from build123d import *

# Parameters (mm, degrees)
RESSALTO_EXTRUS_O2_DEPTH = 9.2
ESBO_O5_R                = 2.15
CORTE_EXTRUS_O2_DEPTH    = 9.2
CHANFRO2_SIZE            = 0.3
SKETCH1_W                = 40
SKETCH1_H                = 3.972261678
BOSS_EXTRUDE1_DEPTH      = 88.9


with BuildPart() as part:
    # Esboço4 → Ressalto-extrusão2 (new body)
    with BuildSketch(Plane(origin=(0, 0, 0), x_dir=(1, 0, 0), z_dir=(0, 1, 0))):
        with BuildLine():
            Line((-19.2, 2.35), (-19.2, 1.65))
            ThreePointArc((-19.2, 1.65), (-19.170710678, 1.579289322), (-19.1, 1.55))
            Line((-19.1, 1.55), (-18.1, 1.55))
            ThreePointArc((-18.1, 1.55), (-18.029289322, 1.579289322), (-18, 1.65))
            Line((-18, 1.65), (-18, 2.35))
            ThreePointArc((-18, 2.35), (-17.970710678, 2.420710678), (-17.9, 2.45))
            Line((-17.9, 2.45), (-17.3, 2.45))
            ThreePointArc((-17.3, 2.45), (-17.229289322, 2.420710678), (-17.2, 2.35))
            Line((-17.2, 2.35), (-17.2, 1.65))
            ThreePointArc((-17.2, 1.65), (-17.170710678, 1.579289322), (-17.1, 1.55))
            Line((-17.1, 1.55), (-16.1, 1.55))
            ThreePointArc((-16.1, 1.55), (-16.029289322, 1.579289322), (-16, 1.65))
            Line((-16, 1.65), (-16, 2.35))
            ThreePointArc((-16, 2.35), (-15.970710678, 2.420710678), (-15.9, 2.45))
            Line((-15.9, 2.45), (-15.3, 2.45))
            ThreePointArc((-15.3, 2.45), (-15.229289322, 2.420710678), (-15.2, 2.35))
            Line((-15.2, 2.35), (-15.2, 1.65))
            ThreePointArc((-15.2, 1.65), (-15.170710678, 1.579289322), (-15.1, 1.55))
            Line((-15.1, 1.55), (-14.1, 1.55))
            ThreePointArc((-14.1, 1.55), (-14.029289322, 1.579289322), (-14, 1.65))
            Line((-14, 1.65), (-14, 2.35))
            ThreePointArc((-14, 2.35), (-13.970710678, 2.420710678), (-13.9, 2.45))
            Line((-13.9, 2.45), (-13.3, 2.45))
            ThreePointArc((-13.3, 2.45), (-13.229289322, 2.420710678), (-13.2, 2.35))
            Line((-13.2, 2.35), (-13.2, 1.65))
            ThreePointArc((-13.2, 1.65), (-13.170710678, 1.579289322), (-13.1, 1.55))
            Line((-13.1, 1.55), (-12.1, 1.55))
            ThreePointArc((-12.1, 1.55), (-12.029289322, 1.579289322), (-12, 1.65))
            Line((-12, 1.65), (-12, 2.35))
            ThreePointArc((-12, 2.35), (-11.970710678, 2.420710678), (-11.9, 2.45))
            Line((-11.9, 2.45), (-11.3, 2.45))
            ThreePointArc((-11.3, 2.45), (-11.229289322, 2.420710678), (-11.2, 2.35))
            Line((-11.2, 2.35), (-11.2, 1.65))
            ThreePointArc((-11.2, 1.65), (-11.170710678, 1.579289322), (-11.1, 1.55))
            Line((-11.1, 1.55), (-10.1, 1.55))
            ThreePointArc((-10.1, 1.55), (-10.029289322, 1.579289322), (-10, 1.65))
            Line((-10, 1.65), (-10, 2.35))
            ThreePointArc((-10, 2.35), (-9.970710678, 2.420710678), (-9.9, 2.45))
            Line((-9.9, 2.45), (-9.3, 2.45))
            ThreePointArc((-9.3, 2.45), (-9.229289322, 2.420710678), (-9.2, 2.35))
            Line((-9.2, 2.35), (-9.2, 1.65))
            ThreePointArc((-9.2, 1.65), (-9.170710678, 1.579289322), (-9.1, 1.55))
            Line((-9.1, 1.55), (-8.1, 1.55))
            ThreePointArc((-8.1, 1.55), (-8.029289322, 1.579289322), (-8, 1.65))
            Line((-8, 1.65), (-8, 2.35))
            ThreePointArc((-8, 2.35), (-7.970710678, 2.420710678), (-7.9, 2.45))
            Line((-7.9, 2.45), (-7.3, 2.45))
            ThreePointArc((-7.3, 2.45), (-7.229289322, 2.420710678), (-7.2, 2.35))
            Line((-7.2, 2.35), (-7.2, 1.65))
            ThreePointArc((-7.2, 1.65), (-7.170710678, 1.579289322), (-7.1, 1.55))
            Line((-7.1, 1.55), (7.1, 1.55))
            ThreePointArc((7.1, 1.55), (7.170710678, 1.579289322), (7.2, 1.65))
            Line((7.2, 1.65), (7.2, 2.35))
            ThreePointArc((7.2, 2.35), (7.229289322, 2.420710678), (7.3, 2.45))
            Line((7.3, 2.45), (7.9, 2.45))
            ThreePointArc((7.9, 2.45), (7.970710678, 2.420710678), (8, 2.35))
            Line((8, 2.35), (8, 1.65))
            ThreePointArc((8, 1.65), (8.029289322, 1.579289322), (8.1, 1.55))
            Line((8.1, 1.55), (9.1, 1.55))
            ThreePointArc((9.1, 1.55), (9.170710678, 1.579289322), (9.2, 1.65))
            Line((9.2, 1.65), (9.2, 2.35))
            ThreePointArc((9.2, 2.35), (9.229289322, 2.420710678), (9.3, 2.45))
            Line((9.3, 2.45), (9.9, 2.45))
            ThreePointArc((9.9, 2.45), (9.970710678, 2.420710678), (10, 2.35))
            Line((10, 2.35), (10, 1.65))
            ThreePointArc((10, 1.65), (10.029289322, 1.579289322), (10.1, 1.55))
            Line((10.1, 1.55), (11.1, 1.55))
            ThreePointArc((11.1, 1.55), (11.170710678, 1.579289322), (11.2, 1.65))
            Line((11.2, 1.65), (11.2, 2.35))
            ThreePointArc((11.2, 2.35), (11.229289322, 2.420710678), (11.3, 2.45))
            Line((11.3, 2.45), (11.9, 2.45))
            ThreePointArc((11.9, 2.45), (11.970710678, 2.420710678), (12, 2.35))
            Line((12, 2.35), (12, 1.65))
            ThreePointArc((12, 1.65), (12.029289322, 1.579289322), (12.1, 1.55))
            Line((12.1, 1.55), (13.1, 1.55))
            ThreePointArc((13.1, 1.55), (13.170710678, 1.579289322), (13.2, 1.65))
            Line((13.2, 1.65), (13.2, 2.35))
            ThreePointArc((13.2, 2.35), (13.229289322, 2.420710678), (13.3, 2.45))
            Line((13.3, 2.45), (13.9, 2.45))
            ThreePointArc((13.9, 2.45), (13.970710678, 2.420710678), (14, 2.35))
            Line((14, 2.35), (14, 1.65))
            ThreePointArc((14, 1.65), (14.029289322, 1.579289322), (14.1, 1.55))
            Line((14.1, 1.55), (15.1, 1.55))
            ThreePointArc((15.1, 1.55), (15.170710678, 1.579289322), (15.2, 1.65))
            Line((15.2, 1.65), (15.2, 2.35))
            ThreePointArc((15.2, 2.35), (15.229289322, 2.420710678), (15.3, 2.45))
            Line((15.3, 2.45), (15.9, 2.45))
            ThreePointArc((15.9, 2.45), (15.970710678, 2.420710678), (16, 2.35))
            Line((16, 2.35), (16, 1.65))
            ThreePointArc((16, 1.65), (16.029289322, 1.579289322), (16.1, 1.55))
            Line((16.1, 1.55), (17.1, 1.55))
            ThreePointArc((17.1, 1.55), (17.170710678, 1.579289322), (17.2, 1.65))
            Line((17.2, 1.65), (17.2, 2.35))
            ThreePointArc((17.2, 2.35), (17.229289322, 2.420710678), (17.3, 2.45))
            Line((17.3, 2.45), (17.9, 2.45))
            ThreePointArc((17.9, 2.45), (17.970710678, 2.420710678), (18, 2.35))
            Line((18, 2.35), (18, 1.65))
            ThreePointArc((18, 1.65), (18.029289322, 1.579289322), (18.1, 1.55))
            Line((18.1, 1.55), (19.1, 1.55))
            ThreePointArc((19.1, 1.55), (19.170710678, 1.579289322), (19.2, 1.65))
            Line((19.2, 1.65), (19.2, 2.35))
            ThreePointArc((19.2, 2.35), (19.229289322, 2.420710678), (19.3, 2.45))
            Line((19.3, 2.45), (19.9, 2.45))
            ThreePointArc((19.9, 2.45), (19.970710678, 2.420710678), (20, 2.35))
            Line((20, 2.35), (20, -2.45))
            Line((20, -2.45), (-20, -2.45))
            Line((-20, -2.45), (-20, 2.35))
            ThreePointArc((-20, 2.35), (-19.970710678, 2.420710678), (-19.9, 2.45))
            Line((-19.9, 2.45), (-19.3, 2.45))
            ThreePointArc((-19.3, 2.45), (-19.229289322, 2.420710678), (-19.2, 2.35))
        make_face()
    extrude(amount=RESSALTO_EXTRUS_O2_DEPTH)

    # Esboço5 → Corte-extrusão2 (cut)
    with BuildSketch(Plane(origin=(0, 0, -1.55), x_dir=(-1, 0, 0), z_dir=(0, 0, -1))):
        with Locations((0, 4.6)):
            Circle(ESBO_O5_R)
    extrude(amount=-CORTE_EXTRUS_O2_DEPTH, mode=Mode.SUBTRACT)

    # Chanfro2
    chanfro2_edges = [part.edges().sort_by_distance(p)[0] for p in [
        (2.15, 4.6, -1.55),
    ]]
    chamfer(chanfro2_edges, length=CHANFRO2_SIZE)

    # Sketch1 → Boss-Extrude1 (add)
    with BuildSketch(Plane.XZ):
        with Locations((0, 0.463869161)):
            Rectangle(SKETCH1_W, SKETCH1_H)
    extrude(amount=BOSS_EXTRUDE1_DEPTH)


solid = part.part
CAD build for the part. Positions are in the model's coordinates, mm. A direction names the side the tool comes from. Give positions to 0.01 mm unless a question says otherwise; leave off trailing zeros. Write each loop counter-clockwise with the first axis right and the second up, starting at its lowest first coordinate (ties: lowest second). Pieces come first, ordered by that corner, then holes. Notation, with made-up numbers: M 71,83 L 84,83 A20 ccw 84,106 Z; hole C 14,47.5 d8. An arc over 180 degrees is marked long. Put each result on its own line as item: value. Start each with the question number.
(1) Mould opens along X. For faces 1 (the face through (0.47, 2.5, 0.57)), 2 (the face through (-20, -39, 1)), 3 (the face through (0, -39, 2.45)) say: +X half, -X half, draft (parallel to the pull), parting line (faces both ways), or undercut.
(2) Band-saw the part on B-B, the plane y = -56.5. Write the cut outline in (x, z), and give its area (3 significant figures).
(3) Which spindle directions (+Z, -Z, +X, -X, +Y, -Y) get a long thin tool onto all of the face, cutting with end or side? Do faces 4 (the face through (0, -44, -1.522)), 5 (the face through (0, 9.2, 1)), 6 (the face through (-2, 7, -1.55)). Say none if no direction does.
(4) Flat gauge pins, fed straight in: pin 1 Ø8 at (x, y) = (-9, -40.5) entering from -Z; pin 2 Ø0.8 at (x, y) = (18.5, 4) entering from -Z; pin 3 Ø0.7 at (x, z) = (-7.5, -2) entering from -Y; pin 4 Ø2.5 at (x, y) = (0, 4.6) entering from -Z. Where does each tip first touch, or does it go through?
(5) Probe L1, parallel to Y at x = 0, z = 1.1; L2, parallel to Z at x = 16, y = -66.5; L3, parallel to X at y = 5, z = 1.9. List the from-to ranges inside material, lowest first.
Response values:
1. face 1: undercut
1. face 2: -X half
1. face 3: draft
2. outline: M -20,-1.52 L 20,-1.52 L 20,2.45 L -20,2.45 Z
2. area: 159 mm2
3. face 4: -Z, +X, -X, -Y
3. face 5: +Z, -Z, +X, -X, +Y
3. face 6: -Z, +Y, -Y
4. pin 1: stops at z = -1.52
4. pin 2: stops at z = -1.55
4. pin 3: stops at y = 0
4. pin 4: passes through
5. L1: y = -88.9 to 2.45, 6.75 to 9.2
5. L2: z = -1.52 to 2.45
5. L3: x = -20 to -2.11, 2.11 to 20
